Here's the drawing with two shaded views (mm, measured from the low corner). I have some questions. Coordinates: 2 decimals unless noted, no trailing zeros. Order: outer loops, then holes, each group sorted by start corner. A loop starts at its lowest first (then second) coordinate and runs counter-clockwise, first axis right, second up. Notation, with made-up numbers: (61, 75.5) -> (95, 75.5) arc R32 ccw to (95, 113.5) -> close; hole circle Ø5 at (-6, 84). An arc over 180 degrees is marked (long way). Return JSON: item names as keys, results as strings. Group by question number.
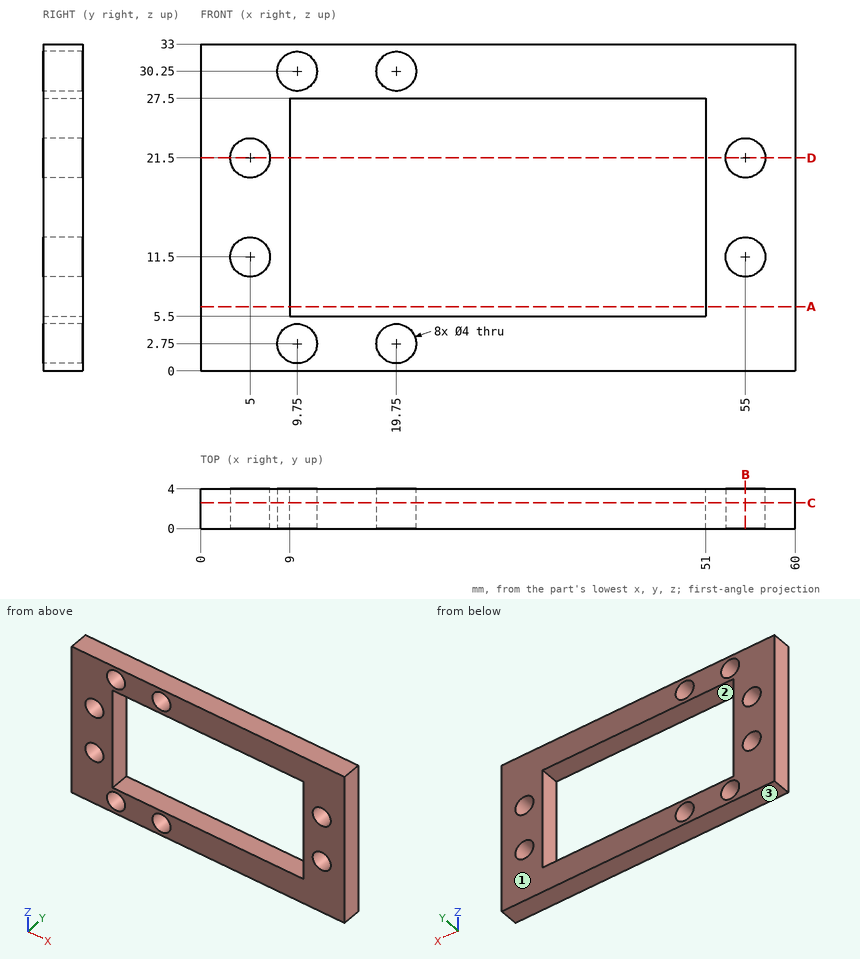
Q1. I need wall thicknesses on line 1 along X through (y, z) = (1.5, 30.25); line 2 along X through (y, z) = (1.1, 21.5); line 3 along Z through (x, y) = (9.75, 2.3). Which ranges of each line are inside material? Lowest first, please. Write a range as from..to.
Q2. We'd pull the mould along Z, two halves only. Please class the marked faces 1, 2 and 3: pulls with the +Z half, pulls with the -Z half, needs draft (parallel to the pull), parting line crosses it, or undercut.
Q3. I want a section at A-A on z = 6.5. Please give me the cut outline in (x, y), and give its area (3 significant figures).
Q4. I want a section at C-C on y = 2.6. State how many separate pieces and enclosed holes the cut face has, and give its area (3 significant figures).
Q5. I want a section at D-D on z = 21.5. Please give me the cut outline in (x, y).
Q6. I want a section at B-B on x = 55. Please give me the cut outline in (y, z), and give its area (3 significant figures).
Q7. I'm going to push a flat-ended pin straight in: pin 1 Ø2.5 at (x, z) = (9.75, 30.25) entering from +Y. Where does the tip first touch, or does it pass through?
Response values:
{
 "1": {"line 1": "x = 0..7.75, 11.75..17.75, 21.75..60", "line 2": "x = 0..3, 7..9, 51..53, 57..60", "line 3": "z = 0..0.75, 4.75..5.5, 27.5..28.25, 32.25..33"},
 "2": {"face 1": "needs draft", "face 2": "undercut", "face 3": "pulls with the -Z half"},
 "3": {"outline": "(0, 0) -> (9, 0) -> (9, 4) -> (0, 4) -> close; (51, 0) -> (60, 0) -> (60, 4) -> (51, 4) -> close", "area": "72.0 mm²"},
 "4": {"separate pieces": "1", "enclosed holes": "9", "area": "955 mm²"},
 "5": {"outline": "(0, 0) -> (3, 0) -> (3, 4) -> (0, 4) -> close; (7, 0) -> (9, 0) -> (9, 4) -> (7, 4) -> close; (51, 0) -> (53, 0) -> (53, 4) -> (51, 4) -> close; (57, 0) -> (60, 0) -> (60, 4) -> (57, 4) -> close"},
 "6": {"outline": "(0, 0) -> (4, 0) -> (4, 9.5) -> (0, 9.5) -> close; (0, 13.5) -> (4, 13.5) -> (4, 19.5) -> (0, 19.5) -> close; (0, 23.5) -> (4, 23.5) -> (4, 33) -> (0, 33) -> close", "area": "100 mm²"},
 "7": {"pin 1": "passes through"}
}
